Geometry check sheet. Reference: drawing and pictorial views, mm from the part's lowest x, y, z. Coordinates: 2 decimals unless noted, no trailing zeros. Write each loop counter-clockwise with the first axis right and the second up, starting at its lowest first coordinate (ties: lowest second). Pieces come first, ordered by that corner, then holes. Notation, with made-up numbers: (74, 34) - (79, 34) arc R24 ccw to (79, 67) - close; hole circle Ø8 at (78.5, -22.75). An arc over 180 degrees is marked (long way). Answer as a JSON object with one key per item and string values. Group by question number.
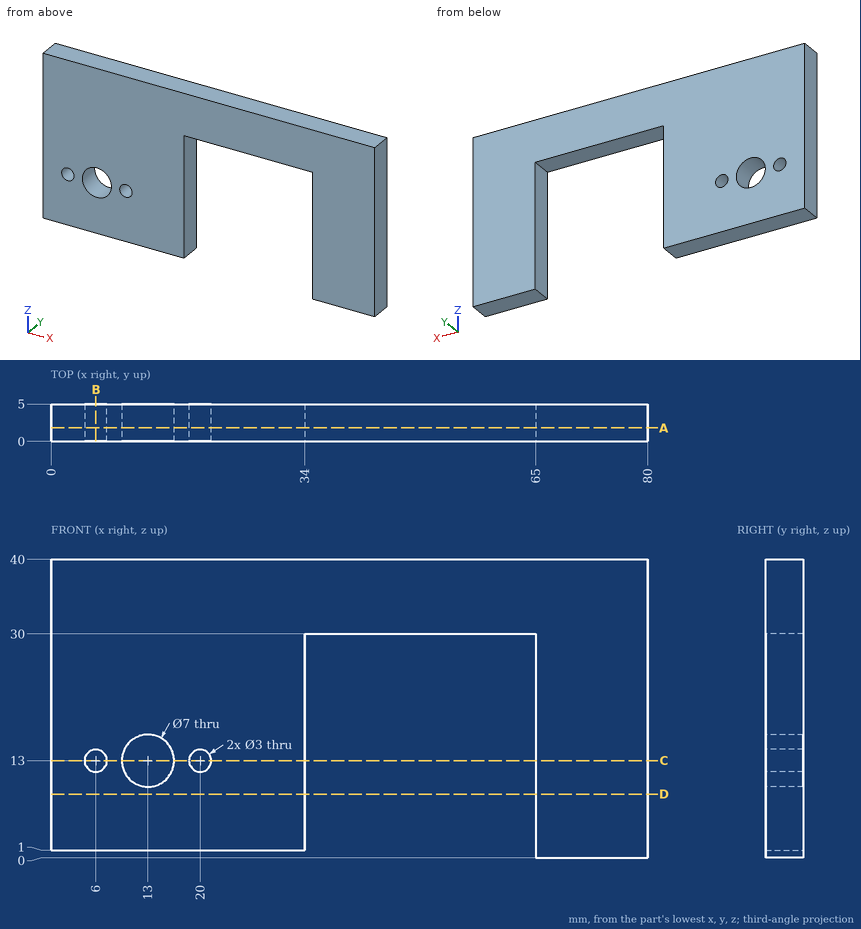
(1) Section check B-B (x = 6). Record the cut outline in (y, z), and give its area (3 significant figures).
(2) Section check C-C (z = 13). Record the cut outline in (x, y), and give its area (3 significant figures).
(3) Material ranges on L1, parallel to Z at x = 6, y = 2.3; L2, parallel to X at y = 4.65, z = 17.5; L3, parallel to X at y = 3, z = 11, recorded low to high. Write a range as [from, to].
(4) Section check A-A (y = 1.8). Record the cut outline in (x, z).
(5) Gauge pin test, flat end, axial feed: pin 1 (2.5 mm diameter, centred on x = 56.5, y = 2, fed in from -Z). Record the tip position at first contact, or that the pin passes through.
(6) Section check D-D (z = 8.5). Record the cut outline in (x, y), and give its area (3 significant figures).
Conclusion:
{
 "1": {"outline": "(0, 1) - (5, 1) - (5, 11.5) - (0, 11.5) - close; (0, 14.5) - (5, 14.5) - (5, 40) - (0, 40) - close", "area": "180 mm^2"},
 "2": {"outline": "(0, 0) - (4.5, 0) - (4.5, 5) - (0, 5) - close; (7.5, 0) - (9.5, 0) - (9.5, 5) - (7.5, 5) - close; (16.5, 0) - (18.5, 0) - (18.5, 5) - (16.5, 5) - close; (21.5, 0) - (34, 0) - (34, 5) - (21.5, 5) - close; (65, 0) - (80, 0) - (80, 5) - (65, 5) - close", "area": "180 mm^2"},
 "3": {"L1": "z = [1, 11.5], [14.5, 40]", "L2": "x = [0, 34], [65, 80]", "L3": "x = [0, 10.13], [15.87, 34], [65, 80]"},
 "4": {"outline": "(0, 1) - (34, 1) - (34, 30) - (65, 30) - (65, 0) - (80, 0) - (80, 40) - (0, 40) - close; hole circle Ø3 at (6, 13); hole circle Ø7 at (13, 13); hole circle Ø3 at (20, 13)"},
 "5": {"pin 1": "stops at z = 30"},
 "6": {"outline": "(0, 0) - (34, 0) - (34, 5) - (0, 5) - close; (65, 0) - (80, 0) - (80, 5) - (65, 5) - close", "area": "245 mm^2"}
}
